from build123d import *

# Parameters (mm, degrees)
F1_ANGLE = -180
F2_R     = 5.08
F3_R     = 2.54


with BuildPart() as f1:
    # F0 (on Front) → F1 (revolve)
    with BuildSketch(Plane.XZ):
        Polygon((133.35, 46.99), (-133.35, 46.99), (-133.35, 6.35), (-120.65, 6.35), (-104.518833, 34.29), (133.35, 34.29), align=None)
    revolve(axis=Axis((1.08064, 0, 0), (1, 0, 0)), revolution_arc=F1_ANGLE)

    # F2
    f2_edges = [f1.edges().sort_by_distance(p)[0] for p in [
        (-133.35, 46.99, 0),
    ]]
    fillet(f2_edges, radius=F2_R)

    # F3
    f3_edges = [f1.edges().sort_by_distance(p)[0] for p in [
        (-133.35, 6.35, 0),
    ]]
    fillet(f3_edges, radius=F3_R)


solid = f1.part
Input: part model. Units: mm. Frame: model coordinates. Round coordinates to 2 decimals unless told otherwise and drop trailing zeros. Write each loop counter-clockwise with the first axis right and the second up, starting at its lowest first coordinate (ties: lowest second). Pieces come first, ordered by that corner, then holes.
1) Draft query along Z for faces 1 (the flat face through (-32, 0, -36)), 2 (the cylindrical face through (16.08, 34.28, 0.75)), 3 (the cylindrical face through (0.71, 46.98, 1.03)). Return one class per face: pulls with the +Z half, pulls with the -Z half, needs draft (parallel to the pull), parting line crosses it, or undercut.
2) Cut plane A-A (z = 0). Return the cut outline in (x, y).
3) Ray query, L1, parallel to Z at x = -105, y = 13; L2, parallel to Z at x = -14, y = 21; L3, parallel to Y at x = -9.5, z = 2.5. Return the intervals inside material, ascending.
4) Cut plane B-B (x = 56). Return the cut outline in (y, z).
5) Contact query for flat-ended pins moving along their axis: P1, Ø10, axis at x = 41, z = 18.5, coming from the +Y side; P2, Ø8, axis at x = -28, y = 31, coming from the +Z side; P3, Ø4, axis at x = 38.5, z = -31, coming from the +Y side. Output: stop coordinate, or through.
Geometry says:
1. face 1: needs draft
1. face 2: undercut
1. face 3: parting line crosses it
2. outline: (-133.35, 8.89) arc R2.54 ccw to (-130.81, 6.35) - (-120.65, 6.35) - (-104.52, 34.29) - (133.35, 34.29) - (133.35, 46.99) - (-128.27, 46.99) arc R5.08 ccw to (-133.35, 41.91) - close
3. L1: z = -45.16 to -30.83, 30.83 to 45.16
3. L2: z = -42.04 to -27.11, 27.11 to 42.04
3. L3: y = 34.2 to 46.92
4. outline: (0, -46.99) arc R46.99 ccw to (0, 46.99) - (0, 34.29) arc R34.29 cw to (0, -34.29) - close
5. P1: stops at y = 45.01
5. P2: stops at z = 38.46
5. P3: stops at y = 36.97
